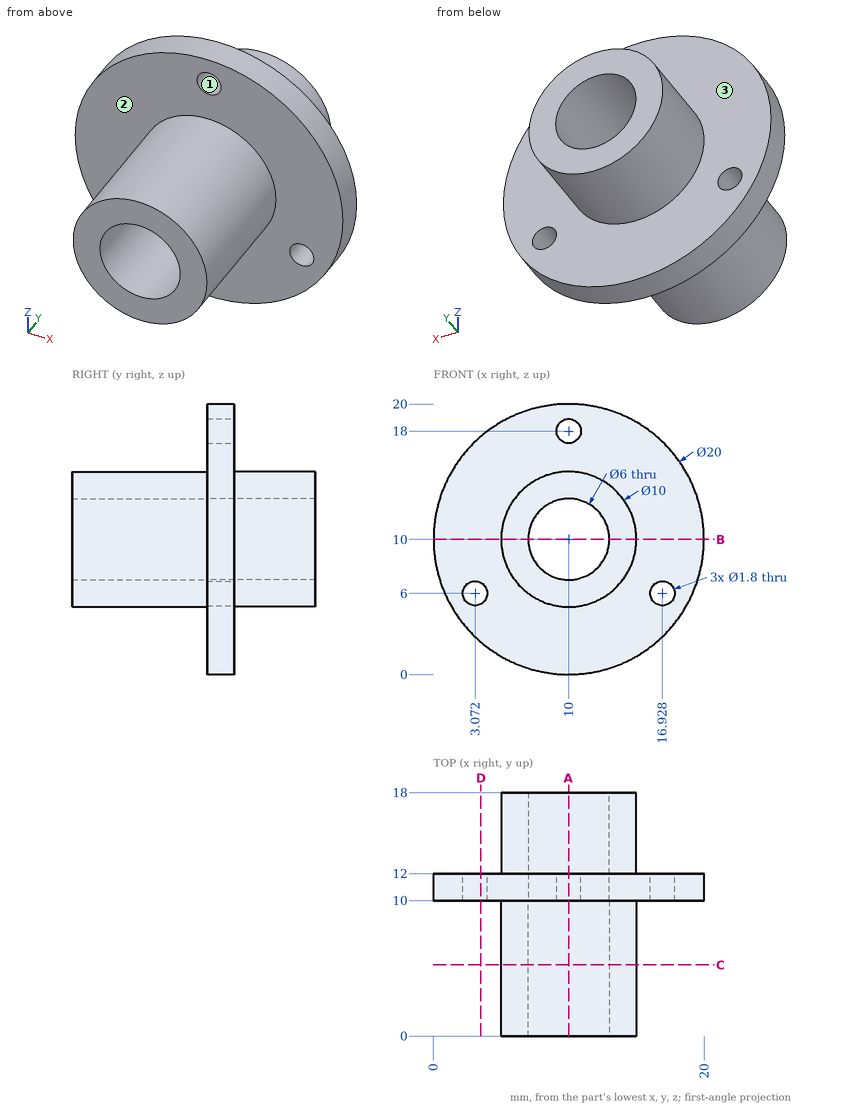
Geometry: see drawing. Coordinates: mm, zero at the bounding-box minimum. A direction names the side the tool comes from. Give positions to 0.01 mm unless a question says otherwise; leave off trailing zeros. Loops run counter-clockwise (first coordinate to the right, second up) from the corner with the lowest first, then second, coordinate; pieces in that order, holes last. Notation, with made-up numbers: (57.25, 42.25) - (82.25, 42.25) arc R6 ccw to (82.25, 46.25) - close; hole circle Ø1 at (-27, 10.5). An arc over 180 degrees is marked (long way). Use CSV: the item, a comma, the result in double quotes. Start each with the question number.
1. Section D-D (x = 3.5). Output: boundary loops of the cut face in (y, z), then the cut area to 3 significant figures.
2. Reachability of the marked faces 1, 2 and 3 from +Z, -Z, +X, -X, +Y, -Y: full face, straight path, thin tool, end or side. Return the list, or none.
3. Section B-B (z = 10). Output: boundary loops of the cut face in (x, y).
4. Pin query (flat end, axial travel): pin 1 (1.6 mm diameter, centred on x = 3.07, z = 6, fed in from -Y); pin 2 (2.5 mm diameter, centred on x = 10, z = 18, fed in from -Y); pin 3 (10 mm diameter, centred on x = 11, z = 15, fed in from -Y); pin 4 (8 mm diameter, centred on y = 15, z = 15, fed in from +X). Return the tip coordinate at first contact, or that it passes through.
5. Ray query, L1, parallel to Z at x = 10, y = 10.7; L2, parallel to Z at x = 10, y = 6.25; L3, parallel to Y at x = 16.75, z = 7.75. Return the intervals inside material, ascending.
6. Section C-C (y = 5.25). Output: boundary loops of the cut face in (x, z).
7. Section A-A (x = 10). Output: boundary loops of the cut face in (y, z).
Response:
1,outline,"(10, 2.4) - (12, 2.4) - (12, 5.21) - (10, 5.21) - close; (10, 6.79) - (12, 6.79) - (12, 17.6) - (10, 17.6) - close"
1,area,"27.2 mm²"
2,face 1,"+Y, -Y"
2,face 2,"-Y"
2,face 3,"+Y"
3,outline,"(0, 10) - (5, 10) - (5, 0) - (7, 0) - (7, 18) - (5, 18) - (5, 12) - (0, 12) - close; (13, 0) - (15, 0) - (15, 10) - (20, 10) - (20, 12) - (15, 12) - (15, 18) - (13, 18) - close"
4,pin 1,"through"
4,pin 2,"y = 10"
4,pin 3,"y = 0"
4,pin 4,"x = 19.72"
5,L1,"0 to 7, 13 to 17.1, 18.9 to 20"
5,L2,"5 to 7, 13 to 15"
5,L3,"10 to 12"
6,outline,"circle Ø10 at (10, 10); hole circle Ø6 at (10, 10)"
7,outline,"(0, 5) - (10, 5) - (10, 0) - (12, 0) - (12, 5) - (18, 5) - (18, 7) - (0, 7) - close; (0, 13) - (18, 13) - (18, 15) - (12, 15) - (12, 17.1) - (10, 17.1) - (10, 15) - (0, 15) - close; (10, 18.9) - (12, 18.9) - (12, 20) - (10, 20) - close"
